Build history of the part. All positions in model axes, mm. Round coordinates to 2 decimals unless told otherwise and drop trailing zeros. Write each loop counter-clockwise with the first axis right and the second up, starting at its lowest first coordinate (ties: lowest second). Pieces come first, ordered by that corner, then holes. Notation, with made-up numbers: (15, -39) -> (72, -39) arc R9 cw to (72, -25) -> close; hole circle Ø11 at (63, 80). An arc over 180 degrees is marked (long way). Return JSON: item names as keys, results as strings.
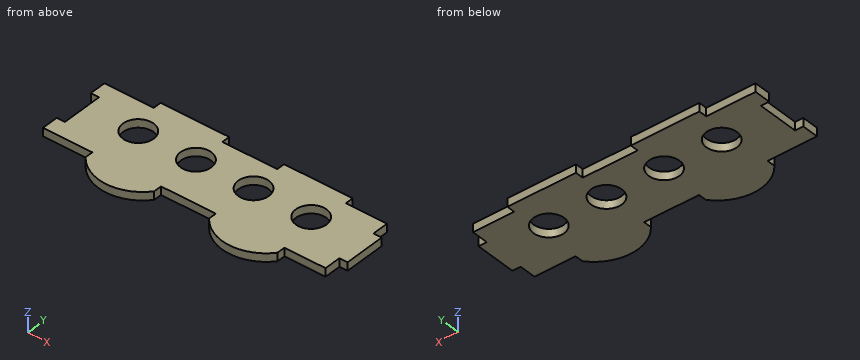
from build123d import *

# Parameters (mm, degrees)
SKETCH_R      = 5.6
EXTRUDE_DEPTH = 3


with BuildPart() as part:
    # Sketch → Extrude (new body)
    with BuildSketch(Plane.XY):
        with BuildLine():
            Line((40, -6.37), (40, -9.37))
            ThreePointArc((15, -9.37), (27.5, -15.37), (40, -9.37))
            Line((15, -9.37), (15, -6.37))
            Line((15, -6.37), (0, -6.37))
            Line((-3, -6.37), (0, -6.37))
            Line((-3, -0.34), (-3, -6.37))
            Line((-3, -0.34), (0, -0.34))
            Line((0, 14.66), (0, -0.34))
            Line((0, 14.66), (-3, 14.66))
            Line((-3, 14.66), (-3, 20.66))
            Line((-3, 20.66), (0, 20.66))
            Line((0, 20.66), (15, 20.66))
            Line((15, 23.66), (15, 20.66))
            Line((40, 23.66), (15, 23.66))
            Line((40, 20.66), (40, 23.66))
            Line((40, 20.66), (60, 20.66))
            Line((60, 23.66), (60, 20.66))
            Line((85, 23.66), (60, 23.66))
            Line((85, 20.66), (85, 23.66))
            Line((85, 20.66), (100, 20.66))
            Line((100, 20.66), (100, 14.66))
            Line((100, 14.66), (103, 14.66))
            Line((103, 14.66), (103, -0.34))
            Line((103, -0.34), (100, -0.34))
            Line((100, -0.34), (100, -6.37))
            Line((100, -6.37), (85, -6.37))
            Line((85, -6.37), (85, -9.37))
            ThreePointArc((60, -9.37), (72.5, -15.37), (85, -9.37))
            Line((60, -9.37), (60, -6.37))
            Line((60, -6.37), (40, -6.37))
        make_face()
        with Locations((18.6, 9.5)):
            Circle(SKETCH_R, mode=Mode.SUBTRACT)
        with Locations((39.6, 9.5)):
            Circle(SKETCH_R, mode=Mode.SUBTRACT)
        with Locations((60.6, 9.5)):
            Circle(SKETCH_R, mode=Mode.SUBTRACT)
        with Locations((81.6, 9.5)):
            Circle(SKETCH_R, mode=Mode.SUBTRACT)
    extrude(amount=EXTRUDE_DEPTH)


solid = part.part
Q1. Saw through at C-C on y = 13. List the corners of the cut face in (x, z), then the cut area to 3 significant figures.
Verdict:
{"outline": "(0, 0) -> (14.23, 0) -> (14.23, 3) -> (0, 3) -> close; (22.97, 0) -> (35.23, 0) -> (35.23, 3) -> (22.97, 3) -> close; (43.97, 0) -> (56.23, 0) -> (56.23, 3) -> (43.97, 3) -> close; (64.97, 0) -> (77.23, 0) -> (77.23, 3) -> (64.97, 3) -> close; (85.97, 0) -> (103, 0) -> (103, 3) -> (85.97, 3) -> close", "area": "204 mm²"}
Q2. Saw through at D-D on x = 18.6. List the corners of the cut face in (y, z), then the cut area to 3 significant figures.
Verdict:
{"outline": "(-12.67, 0) -> (3.9, 0) -> (3.9, 3) -> (-12.67, 3) -> close; (15.1, 0) -> (23.66, 0) -> (23.66, 3) -> (15.1, 3) -> close", "area": "75.4 mm²"}
Q3. Saw through at B-B on x = 36.5. List the corners of the cut face in (y, z).
Verdict:
{"outline": "(-12.6, 0) -> (4.84, 0) -> (4.84, 3) -> (-12.6, 3) -> close; (14.16, 0) -> (23.66, 0) -> (23.66, 3) -> (14.16, 3) -> close"}
Q4. Pin check, flat tips, straight feed: pin 1 Ø0.9 at (x, z) = (50, 2) entering from +Y; pin 2 Ø10 at (x, y) = (18.6, 9.5) entering from +Z; pin 3 Ø1.5 at (y, z) = (-7.5, 1) entering from +X; pin 4 Ø0.9 at (x, z) = (91, 1.5) entering from -Y. Stop position of each tip, or through.
Verdict:
{"pin 1": "stops at y = 20.66", "pin 2": "passes through", "pin 3": "stops at x = 85", "pin 4": "stops at y = -6.37"}
Q5. Saw through at A-A on z = 1.2. Count the separate pieces of the cut face and the enclosed holes in it, then the cut area to 3 significant figures.
Verdict:
{"separate pieces": "1", "enclosed holes": "4", "area": "2,900 mm²"}
Q6. Wall check: L1, parallel to X at y = -8.5, z = 1.45; L2, parallel to X at y = 5.5, z = 2.55; L3, parallel to X at y = 1.5, z = 0.2. Give the ranges that are in metal, low to high.
Verdict:
{"L1": "x = 15 to 40, 60 to 85", "L2": "x = 0 to 14.68, 22.52 to 35.68, 43.52 to 56.68, 64.52 to 77.68, 85.52 to 103", "L3": "x = 0 to 103"}
